The listing builds one solid part. Answer for the finished solid, in the listing's coordinates (mm). A direction names the side the tool comes from. Give positions to 0.01 mm unless a question says otherwise; leave off trailing zeros. Write each loop counter-clockwise with the first axis right and the second up, starting at its lowest first coordinate (ties: lowest second). Pieces come first, ordered by that corner, then holes. Notation, with made-up numbers: M 57.25,17 L 104.25,17 A22 cw 104.25,35 Z; hole C 5.25,60 d6. An arc over 180 degrees is marked long. Return JSON: item names as keys, results as strings.
from build123d import *

# Parameters (mm, degrees)
PRISM_DEPTH = 2.5


with BuildPart() as part:
    # Sketch_002 → Revolution (revolve)
    with BuildSketch(Plane.XY):
        with BuildLine():
            Line((-1.5, 4.161438), (-1.5, 1.75))
            Line((-1.5, 1.75), (0.25, 0))
            Line((0.25, 0), (25, 0))
            Line((25, 0), (25, 1.9))
            Line((25, 1.9), (24.5, 2.4))
            Line((24.5, 2.4), (0, 2.4))
            Line((0, 2.4), (0, 4.161438))
            ThreePointArc((0, 4.161438), (-0.75, 4.5), (-1.5, 4.161438))
        make_face()
    revolve(axis=Axis((0, 0, 0), (1, 0, 0)))

    # Prism → Prism (cut)
    with BuildSketch(Plane(origin=(-1.5, 0, 0), x_dir=(0, 0, 1), z_dir=(1, 0, 0))):
        Polygon((1.732051, 0), (0.866025, 1.5), (-0.866025, 1.5), (-1.732051, 0), (-0.866025, -1.5), (0.866025, -1.5), align=None)
    extrude(amount=PRISM_DEPTH, mode=Mode.SUBTRACT)


solid = part.part
Item 1: Find the intervals of material crossed by line 1 (X direction, y = -2.5, z = 0.75); line 2 (Y direction, x = -0.25, z = 0.5); line 3 (Y direction, x = 23, z = 0.5), in increasing order.
Geometry results:
{"line 1": "x = -1.5 to 0", "line 2": "y = -4.34 to -1.5, 1.5 to 4.34", "line 3": "y = -2.35 to 2.35"}
Item 2: Which of the six approach directions +Z, -Z, +X, -X, +Y, -Y give full straight-line access (tool end or side, diameter ignored) to faces 1 (the flat face through (-1.5, 2, 0)), 2 (the flat face through (0, -2, -2)), 3 (the flat face through (-0.258, 0.76, 1.293))?
Geometry results:
{"face 1": "+Z, -Z, -X, +Y, -Y", "face 2": "+X", "face 3": "-X"}
Item 3: A cutting plane is placed at A-A, the plane z = 0. Write down the section's boundary in (x, y).
Geometry results:
{"outline": "M -1.5,-4.16 A1 ccw 0,-4.16 L 0,-2.4 L 24.5,-2.4 L 25,-1.9 L 25,1.9 L 24.5,2.4 L 0,2.4 L 0,4.16 A1 ccw -1.5,4.16 L -1.5,1.75 L -1.25,1.5 L 1,1.5 L 1,-1.5 L -1.25,-1.5 L -1.5,-1.75 Z"}
Item 4: Determine the mould class of faces 4 (the cylindrical face through (12.078, 1.29, 2.024)), 5 (the flat face through (25, 0, 0)), 6 (the flat face through (0, -1.5, 0)) for opening direction Y: +Y half, -Y half, draft (parallel to the pull), parting line (faces both ways), or undercut.
Geometry results:
{"face 4": "parting line", "face 5": "draft", "face 6": "undercut"}
Item 5: A cutting plane is placed at B-B, the plane x = 22.75. Write down the section's boundary in (y, z), plus the area to 3 significant figures.
Geometry results:
{"outline": "C 0,0 d4.8", "area": "18.1 mm2"}
Item 6: Given pin 1 Ø3.5 at (y, z) = (-0.5, 0.5) entering from -X; pin 2 Ø1.5 at (y, z) = (-0.5, -3) entering from +X; pin 3 Ø0.9 at (x, z) = (0, 0) entering from +Y; pin 4 Ø4 at (x, z) = (9.5, 1.5) entering from +Y, each flat-ended and moving along its own axis, determine where each tip first touches the part or whether it passes through.
Geometry results:
{"pin 1": "stops at x = -1.5", "pin 2": "stops at x = 24.61", "pin 3": "stops at y = 4.45", "pin 4": "stops at y = 2.4"}
